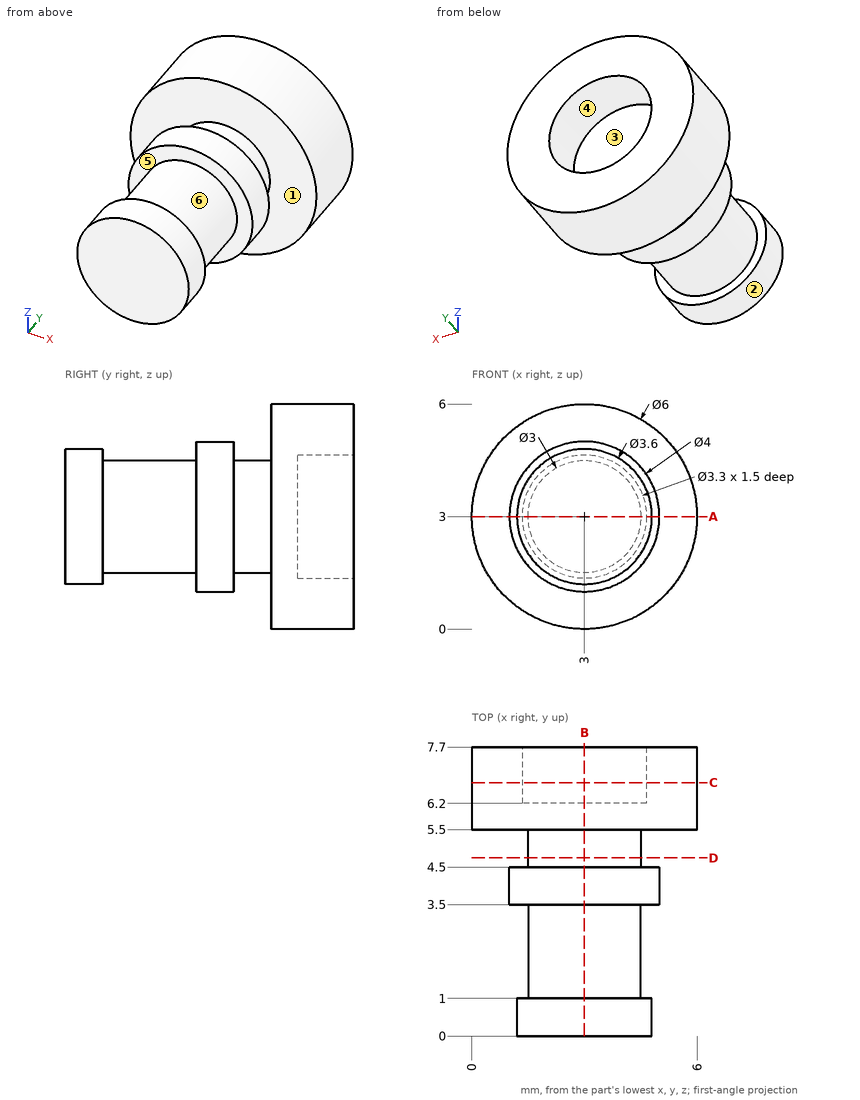
The drawing under review shows one solid part. Ordinate dimensions are in mm from its lowest x, y, z. A direction names the side the tool comes from. Coordinates: 2 decimals unless noted, no trailing zeros. Write each loop counter-clockwise with the first axis right and the second up, starting at its lowest first coordinate (ties: lowest second). Pieces come first, ordered by that corner, then holes. Notation, with made-up numbers: (-26.5, 53) - (-20.5, 53) arc R10 ccw to (-20.5, 68) - close; hole circle Ø5 at (-23, -16.75). An arc over 180 degrees is marked (long way). Answer in a Markdown table with one row per item. Add a question column.
Q1. Tool access review of the marked faces 1, 2 and 3: name each direction out of +Z, -Z, +X, -X, +Y, -Y from which nothing blocks a thin tool from reaching the whole face with its end or side.
Q2. For P1, Ø1, axis at y = 4.5, z = 2.5, coming from the +X side; P2, Ø1.5, axis at x = 2.5, y = 3.5, coming from the -Z side; P3, Ø1.2, axis at x = 2, z = 3, coming from the +Y side, all flat-tipped, find the tip position at first contact; note any pin that passes through.
Q3. We need section A-A, the plane z = 3. State the section outline as (x, y) points, and give its area (4 significant figures).
Q4. We need section B-B, the plane x = 3. State the section outline as (y, z) points, and give its area (4 significant figures).
Q5. We need section C-C, the plane y = 6.75. State the section outline as (x, z) points.
Q6. We need section D-D, the plane y = 4.75. State the section outline as (x, z) points, and give its area (3 significant figures).
Q7. For probe 1 along Y at (x, z) = (1.95, 1.85); probe 2 along X at (y, z) = (7.35, 3); probe 3 along Y at (x, z) = (1.2, 2.65), list the stretches that pass through material, from the lowest coordinate up.
Q8. Draft analysis for pull direction X (two halves, no side actions). For the marked faces 4, 5 and 6, state which applies: +X half, -X half, draft (parallel to the pull), parting line (faces both ways), or undercut.
Answer list:
| question | item | result |
|---|---|---|
| 1 | face 1 | none |
| 1 | face 2 | -Y |
| 1 | face 3 | +Y |
| 2 | P1 | stops at x = 5 |
| 2 | P2 | stops at z = 1 |
| 2 | P3 | stops at y = 6.2 |
| 3 | outline | (0, 5.5) - (1.5, 5.5) - (1.5, 4.5) - (1, 4.5) - (1, 3.5) - (1.5, 3.5) - (1.5, 1) - (1.2, 1) - (1.2, 0) - (4.8, 0) - (4.8, 1) - (4.5, 1) - (4.5, 3.5) - (5, 3.5) - (5, 4.5) - (4.5, 4.5) - (4.5, 5.5) - (6, 5.5) - (6, 7.7) - (4.65, 7.7) - (4.65, 6.2) - (1.35, 6.2) - (1.35, 7.7) - (0, 7.7) - close |
| 3 | area | 26.35 mm2 |
| 4 | outline | (0, 1.2) - (1, 1.2) - (1, 1.5) - (3.5, 1.5) - (3.5, 1) - (4.5, 1) - (4.5, 1.5) - (5.5, 1.5) - (5.5, 0) - (7.7, 0) - (7.7, 1.35) - (6.2, 1.35) - (6.2, 4.65) - (7.7, 4.65) - (7.7, 6) - (5.5, 6) - (5.5, 4.5) - (4.5, 4.5) - (4.5, 5) - (3.5, 5) - (3.5, 4.5) - (1, 4.5) - (1, 4.8) - (0, 4.8) - close |
| 4 | area | 26.35 mm2 |
| 5 | outline | circle Ø6 at (3, 3); hole circle Ø3.3 at (3, 3) |
| 6 | outline | circle Ø3 at (3, 3) |
| 6 | area | 7.07 mm2 |
| 7 | probe 1 | y = 0 to 1, 3.5 to 4.5, 5.5 to 6.2 |
| 7 | probe 2 | x = 0 to 1.35, 4.65 to 6 |
| 7 | probe 3 | y = 3.5 to 4.5, 5.5 to 7.7 |
| 8 | face 4 | undercut |
| 8 | face 5 | draft |
| 8 | face 6 | parting line |
